Read the model definition and answer for the solid it produces. Units are mm, in the model's axes. Give positions to 0.01 mm unless a question says otherwise; leave off trailing zeros. Order: outer loops, then holes, each group sorted by start corner. A loop starts at its lowest first (then second) coordinate and runs counter-clockwise, first axis right, second up. Notation, with made-up numbers: (1, 63) -> (17, 63) arc R23 cw to (17, 101) -> close; hole circle Ø3 at (50.25, 61.5). An arc over 180 degrees is marked (long way). Use one line per item in the form item = value.
```python
from build123d import *

# Parameters (mm, degrees)
BOSS_EXTRUDE1_DEPTH     = 5.08
CUT_EXTRUDE1_DEPTH      = 109.941018249
CUT_EXTRUDE1_DEPTH_BACK = 109.941018249
CUT_EXTRUDE2_DEPTH      = 185.574421805
CUT_EXTRUDE2_DEPTH_BACK = 185.574421805
SKETCH4_R               = 1.905
CUT_EXTRUDE3_DEPTH      = 21.336


with BuildPart() as part:
    # Sketch1 → Boss-Extrude1 (new body)
    with BuildSketch(Plane(origin=(0, 0, 0), x_dir=(1, 0, 0), z_dir=(0, 1, 0))):
        Polygon((7.62, -91.9861), (7.62, 91.9861), (0, 104.6861), (0, -104.6861), align=None)
        Polygon((0, 91.9861), (0, 104.6861), (-22.098, 104.6861), align=None)
    extrude(amount=BOSS_EXTRUDE1_DEPTH)

    # Sketch2 → Cut-Extrude1 (cut, two sides: drawn at the far end of the back side and taken through both)
    with BuildSketch(Plane(origin=(7.62, 0, 0), x_dir=(0, 0, -1), z_dir=(1, 0, 0)).offset(-CUT_EXTRUDE1_DEPTH_BACK)):
        Polygon((-104.6861, 5.08), (-91.9861, 5.08), (-104.6861, 2.54), align=None)
        Polygon((-104.6861, 0), (-104.6861, 2.54), (-91.9861, 0), align=None)
    extrude(amount=CUT_EXTRUDE1_DEPTH + CUT_EXTRUDE1_DEPTH_BACK, mode=Mode.SUBTRACT)

    # Sketch3 → Cut-Extrude2 (cut, two sides: drawn at the far end of the back side and taken through both)
    with BuildSketch(Plane(origin=(39.73974923, 0, -69.147163661), x_dir=(0.867013943985018, 0, 0.4982838758534578), z_dir=(-0.4982838758534578, 0, 0.867013943985018)).offset(-CUT_EXTRUDE2_DEPTH_BACK)):
        Polygon((-71.32266979, 2.54), (-45.835190433, 5.08), (-71.32266979, 5.08), align=None)
        Polygon((-45.835190433, 0), (-71.32266979, 2.54), (-71.32266979, 0), align=None)
    extrude(amount=CUT_EXTRUDE2_DEPTH + CUT_EXTRUDE2_DEPTH_BACK, mode=Mode.SUBTRACT)

    # Sketch4 → Cut-Extrude3 (cut)
    with BuildSketch(Plane.ZY):
        with Locations((-3.3401, 2.54)):
            Circle(SKETCH4_R)
    extrude(amount=-CUT_EXTRUDE3_DEPTH, mode=Mode.SUBTRACT)


solid = part.part
```
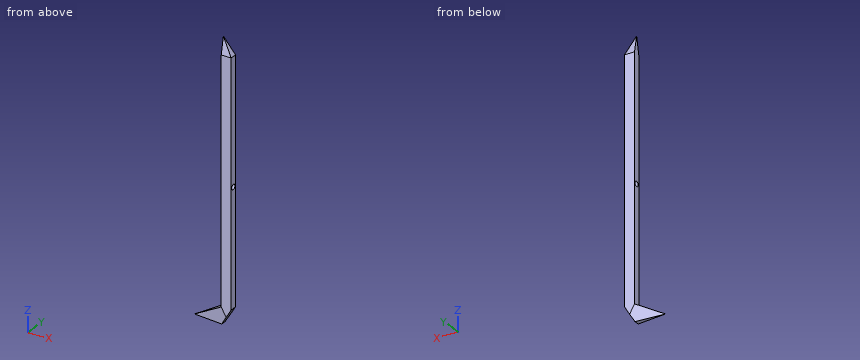
Item 1: Given pin 1 Ø3 at (x, y) = (-10, 1) entering from -Z; pin 2 Ø3 at (x, y) = (1.5, 1) entering from +Z, each flat-ended and moving along its own axis, determine where each tip first touches the part or whether it passes through.
Checks:
pin_1 = -104.69
pin_2 = 103.45
Item 2: The part is cut by section B-B on x = -7.5. Give the vertices of the cut face in (y, z), and give its area (3 significant figures).
Checks:
outline = (0.86, -96.3) -> (1.28, -104.69) -> (3.8, -104.69) -> (4.22, -96.3) -> close
area = 24.7 mm²
Item 3: Straight lines are drawn through the part: L1, parallel to X at y = 4.7, z = -69.5; L2, parallel to X at y = 2.3, z = 95.5; L3, parallel to Z at x = -6, y = 3.05. For each, find the intervals that lie inside material, in ascending order. Write a range as from..to.
Checks:
L1 = 0..7.62
L2 = 0..5.51
L3 = -104.69..-95.43
Item 4: The part is cut by section A-A on z = 56.5. Give the vertices of the cut face in (x, y), and give its area (3 significant figures).
Checks:
outline = (0, 0) -> (7.62, 0) -> (7.62, 5.08) -> (0, 5.08) -> close
area = 38.7 mm²
